For this review, take the finished solid that the model builds, in its own axes (mm). A direction names the side the tool comes from. Coordinates: 2 decimals unless noted, no trailing zeros. Order: outer loops, then holes, each group sorted by start corner. A loop starts at its lowest first (then second) coordinate and runs counter-clockwise, first axis right, second up. Notation, with made-up numbers: (67, 28) -> (101, 28) arc R21 cw to (101, 57) -> close; hole circle Ø7 at (27, -39). An arc over 180 degrees is marked (long way). Return JSON: item names as keys, results as strings. Group by question number.
Item 1: Insertion check: pin 1 (4 mm diameter, centred on x = -53.69, y = -49.12, fed in from +Z); pin 2 (3 mm diameter, centred on x = -53.69, y = -9.12, fed in from +Z); pin 3 (8 mm diameter, centred on x = 54.71, y = -49.12, fed in from -Z); pin 4 (1 mm diameter, centred on y = -7.5, z = 0.5, fed in from -X). Each pin has a flat end and moves straight along its axis. Give the tip position at first contact, or say it passes through.
Item 2: Take a section at C-C (y = -70). Write out the cut boundary in (x, z).
Item 3: Take a section at B-B (y = -15.5). Write out the cut boundary in (x, z).
Item 4: Take a section at A-A (x = -16). Write out the cut boundary in (y, z), then the cut area to 3 significant figures.
Item 5: Machinability: for faces 5 (the flat face through (64.261, -24, 1)), 6 (the cylindrical face through (-38.51, -63.63, 1.27)), 7 (the flat face through (-52, -10, 1)), which of the approach directions +Z, -Z, +X, -X, +Y, -Y give a long, thin tool a straight path to every point of the face, cutting with its end or side? Answer none if there is none.
Item 6: Draft analysis for pull direction Y (two halves, no side actions). For faces 1 (the cylindrical face through (-52.65, -47.78, 0.51)), 2 (the flat face through (1, 40.926, 0)), 3 (the cylindrical face through (-52.35, -88.24, 1.75)), 4 (the flat face through (43, -28, 2.5)), state which applies: +Y half, -Y half, draft (parallel to the pull), parting line (faces both ways), or undercut.
Item 7: For line 1 along Y through (x, z) = (17, 0.1); line 2 along X through (y, z) = (14.5, 0.5); line 3 along X through (y, z) = (-33, 2.05), list the stretches that pass through material, from the lowest coordinate up.
```python
from build123d import *

# Parameters (mm, degrees)
ESBO_O1_W                                      = 130
ESBO_O1_H                                      = 140.05
RESSALTO_EXTRUS_O1_DEPTH                       = 2.5
ESBO_O2_W                                      = 130
ESBO_O2_H                                      = 4
RESSALTO_EXTRUS_O2_DEPTH                       = 2.25
FILETE1_R                                      = 2
ESBO_O3_W                                      = 130
ESBO_O3_H                                      = 1
CORTE_EXTRUS_O1_DEPTH                          = 2
ESBO_O6_W                                      = 1.25
ESBO_O6_H                                      = 140.05
CORTE_EXTRUS_O2_DEPTH                          = 3.5
ESBO_O8_W                                      = 1.25
ESBO_O8_H                                      = 3.5
CORTE_EXTRUS_O3_DEPTH                          = 6.25
REBAIXO_PARA_PARAFUSO_COM_CABE_A_PAN_2_COUNT   = 2
REBAIXO_PARA_PARAFUSO_COM_CABE_A_PAN_2_PITCH   = 40
REBAIXO_PARA_PARAFUSO_COM_CABE_A_PAN_3_COUNT   = 2
REBAIXO_PARA_PARAFUSO_COM_CABE_A_PAN_3_PITCH   = 108.4
REBAIXO_PARA_PARAFUSO_COM_CABE_A_PAN_4_COUNT   = 2
REBAIXO_PARA_PARAFUSO_COM_CABE_A_PAN_4_PITCH   = 115.544623415
CORTE_EXTRUS_O5_DEPTH                          = 8.25
REBAIXO_PARA_PARAFUSO_COM_CABE_A_PAN_5_A_COUNT = 2
REBAIXO_PARA_PARAFUSO_COM_CABE_A_PAN_5_A_PITCH = 101


with BuildPart() as part:
    # Esboço1 → Ressalto-extrusão1 (new body)
    with BuildSketch(Plane.XY):
        with Locations((0.510662177, -29.099074074)):
            Rectangle(ESBO_O1_W, ESBO_O1_H)
    extrude(amount=RESSALTO_EXTRUS_O1_DEPTH)

    # Esboço2 → Ressalto-extrusão2 (add)
    with BuildSketch(Plane(origin=(0, 0, 0), x_dir=(-1, 0, 0), z_dir=(0, 0, -1))):
        with Locations((-0.510662177, 38.925925926)):
            Rectangle(ESBO_O2_W, ESBO_O2_H)
    extrude(amount=RESSALTO_EXTRUS_O2_DEPTH)

    # Filete1
    filete1_edges = [part.edges().sort_by_distance(p)[0] for p in [
        (0.510662177, 36.925925926, 0),
    ]]
    fillet(filete1_edges, radius=FILETE1_R)

    # Esboço3 → Corte-extrusão1 (cut)
    with BuildSketch(Plane(origin=(0, 0, -2.25), x_dir=(-1, 0, 0), z_dir=(0, 0, -1))):
        with Locations((-0.510662177, 38.925925926)):
            Rectangle(ESBO_O3_W, ESBO_O3_H)
    extrude(amount=-CORTE_EXTRUS_O1_DEPTH, mode=Mode.SUBTRACT)

    # Esboço6 → Corte-extrusão2 (cut)
    with BuildSketch(Plane(origin=(0, 0, -2.25), x_dir=(-1, 0, 0), z_dir=(0, 0, -1))):
        with Locations((-64.885662177, -29.099074074)):
            Rectangle(ESBO_O6_W, ESBO_O6_H)
        with Locations((63.864337823, -29.099074074)):
            Rectangle(ESBO_O6_W, ESBO_O6_H)
    extrude(amount=-CORTE_EXTRUS_O2_DEPTH, mode=Mode.SUBTRACT)

    # Esboço8 → Corte-extrusão3 (cut)
    with BuildSketch(Plane(origin=(0, 40.925925926, 0), x_dir=(1, 0, 0), z_dir=(0, 1, 0))):
        with Locations((-62.614337823, 0.5)):
            Rectangle(ESBO_O8_W, ESBO_O8_H)
    extrude(amount=-CORTE_EXTRUS_O3_DEPTH, mode=Mode.SUBTRACT)

    # Esboço12 → Rebaixo para parafuso com cabe_a panela (revolve, cut)
    with BuildSketch(Plane(origin=(-53.689337823, -9.124074074, 2.5), x_dir=(0, -1, 0), z_dir=(1, 0, 0))):
        Polygon((0, 0), (0, 4.75), (1.7, 4.75), (1.7, 1.5), (3.5, 1.5), (3.5, 0.025), (3.525, 0), align=None)
    rebaixo_para_parafuso_com_cabe_a_panela = revolve(axis=Axis((-53.689337823, -9.124074074, 8.85), (0, 0, -1)), mode=Mode.SUBTRACT)

    # Rebaixo para parafuso com cabe_a pan 2: Rebaixo para parafuso com cabe_a panela ×2
    with Locations(*[(0, -i * REBAIXO_PARA_PARAFUSO_COM_CABE_A_PAN_2_PITCH, 0) for i in range(1, REBAIXO_PARA_PARAFUSO_COM_CABE_A_PAN_2_COUNT)]):
        add(rebaixo_para_parafuso_com_cabe_a_panela, mode=Mode.SUBTRACT)

    # Rebaixo para parafuso com cabe_a pan 3: Rebaixo para parafuso com cabe_a panela ×2
    with Locations(*[(i * REBAIXO_PARA_PARAFUSO_COM_CABE_A_PAN_3_PITCH, 0, 0) for i in range(1, REBAIXO_PARA_PARAFUSO_COM_CABE_A_PAN_3_COUNT)]):
        add(rebaixo_para_parafuso_com_cabe_a_panela, mode=Mode.SUBTRACT)

    # Rebaixo para parafuso com cabe_a pan 4: Rebaixo para parafuso com cabe_a panela ×2
    with Locations(*[Vector(0.9381656783035653, -0.3461865971599872, 0) * (i * REBAIXO_PARA_PARAFUSO_COM_CABE_A_PAN_4_PITCH) for i in range(1, REBAIXO_PARA_PARAFUSO_COM_CABE_A_PAN_4_COUNT)]):
        add(rebaixo_para_parafuso_com_cabe_a_panela, mode=Mode.SUBTRACT)

    # Esboço13 → Corte-extrusão5 (cut)
    with BuildSketch(Plane.XY.offset(2.5)):
        with BuildLine():
            Line((32.535999817, -66.48621762), (-31.514675462, -66.48621762))
            ThreePointArc((-31.514675462, -66.48621762), (-38.585743274, -63.557285432), (-41.514675462, -56.48621762))
            Line((-41.514675462, -56.48621762), (-41.514675462, 15.639195022))
            ThreePointArc((-41.514675462, 15.639195022), (-38.585743274, 22.710262834), (-31.514675462, 25.639195022))
            Line((-31.514675462, 25.639195022), (32.535999817, 25.639195022))
            ThreePointArc((32.535999817, 25.639195022), (39.607067629, 22.710262834), (42.535999817, 15.639195022))
            Line((42.535999817, 15.639195022), (42.535999817, -56.48621762))
            ThreePointArc((42.535999817, -56.48621762), (39.607067629, -63.557285432), (32.535999817, -66.48621762))
        make_face()
        with BuildLine():
            Line((34.535999817, -91.70501851), (-33.514675462, -91.70501851))
            ThreePointArc((-33.514675462, -91.70501851), (-39.171529712, -89.361872759), (-41.514675462, -83.70501851))
            Line((-41.514675462, -83.70501851), (-41.514675462, -81.880603518))
            ThreePointArc((-41.514675462, -81.880603518), (-39.171529712, -76.223749269), (-33.514675462, -73.880603518))
            Line((-33.514675462, -73.880603518), (34.535999817, -73.880603518))
            ThreePointArc((34.535999817, -73.880603518), (40.192854066, -76.223749269), (42.535999817, -81.880603518))
            Line((42.535999817, -81.880603518), (42.535999817, -83.70501851))
            ThreePointArc((42.535999817, -83.70501851), (40.192854066, -89.361872759), (34.535999817, -91.70501851))
        make_face()
    extrude(amount=-CORTE_EXTRUS_O5_DEPTH, mode=Mode.SUBTRACT)

    # Esboço16 → Rebaixo para parafuso com cabe_a pan 5 (revolve, cut)
    with BuildSketch(Plane(origin=(-49.989337823, -90.824074074, 2.5), x_dir=(0, -1, 0), z_dir=(1, 0, 0))):
        Polygon((0, 0), (0, 4.75), (1.7, 4.75), (1.7, 1.5), (3.5, 1.5), (3.5, 0.025), (3.525, 0), align=None)
    rebaixo_para_parafuso_com_cabe_a_pan_5 = revolve(axis=Axis((-49.989337823, -90.824074074, 8.85), (0, 0, -1)), mode=Mode.SUBTRACT)

    # Rebaixo para parafuso com cabe_a pan 5 a: Rebaixo para parafuso com cabe_a pan 5 ×2
    with Locations(*[(i * REBAIXO_PARA_PARAFUSO_COM_CABE_A_PAN_5_A_PITCH, 0, 0) for i in range(1, REBAIXO_PARA_PARAFUSO_COM_CABE_A_PAN_5_A_COUNT)]):
        add(rebaixo_para_parafuso_com_cabe_a_pan_5, mode=Mode.SUBTRACT)


solid = part.part
```
Findings below:
{
 "1": {"pin 1": "stops at z = 1", "pin 2": "passes through", "pin 3": "stops at z = 0", "pin 4": "stops at x = -63.24"},
 "2": {"outline": "(-64.49, 1.25) -> (-63.24, 1.25) -> (-63.24, 0) -> (64.26, 0) -> (64.26, 1.25) -> (65.51, 1.25) -> (65.51, 2.5) -> (-64.49, 2.5) -> close"},
 "3": {"outline": "(-64.49, 1.25) -> (-63.24, 1.25) -> (-63.24, 0) -> (-41.51, 0) -> (-41.51, 2.5) -> (-64.49, 2.5) -> close; (42.54, 0) -> (64.26, 0) -> (64.26, 1.25) -> (65.51, 1.25) -> (65.51, 2.5) -> (42.54, 2.5) -> close"},
 "4": {"outline": "(-99.12, 0) -> (-91.71, 0) -> (-91.71, 2.5) -> (-99.12, 2.5) -> close; (-73.88, 0) -> (-66.49, 0) -> (-66.49, 2.5) -> (-73.88, 2.5) -> close; (25.64, 0) -> (34.93, 0) arc R2 cw to (36.93, -2) -> (36.93, -2.25) -> (38.43, -2.25) -> (38.43, -0.25) -> (39.43, -0.25) -> (39.43, -2.25) -> (40.93, -2.25) -> (40.93, 2.5) -> (25.64, 2.5) -> close", "area": "83.1 mm2"},
 "5": {"face 5": "-Z, +X, +Y, -Y", "face 6": "+Z, -Z", "face 7": "+Z"},
 "6": {"face 1": "undercut", "face 2": "+Y half", "face 3": "undercut", "face 4": "draft"},
 "7": {"line 1": "y = -99.12 to -91.71, -73.88 to -66.49, 25.64 to 40.93", "line 2": "x = -63.24 to -41.51, 42.54 to 64.26", "line 3": "x = -64.49 to -41.51, 42.54 to 65.51"}
}
